Build history of the part. All positions in model axes, mm. Face numbers are marked on the shaded views. A direction names the side the tool comes from. Coordinates: 2 decimals unless noted, no trailing zeros. Order: outer loops, then holes, each group sorted by start corner. A loop starts at its lowest first (then second) coordinate and runs counter-clockwise, first axis right, second up. Notation, with made-up numbers: (43, -31) - (56, -31) arc R31 ccw to (56, -6) - close; hole circle Ø7 at (-39, -24.5). An arc over 180 degrees is marked (long way). One line per item, written item: value.
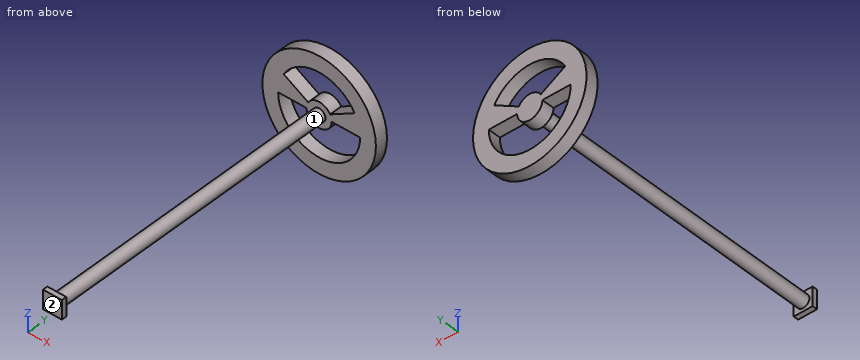
from build123d import *

# Parameters (mm, degrees)
SKETCH1_W           = 38.1
SKETCH1_H           = 38.1
BOSS_EXTRUDE1_DEPTH = 10
SKETCH2_R           = 12.7
BOSS_EXTRUDE2_DEPTH = 600
SKETCH3_R           = 114.3
BOSS_EXTRUDE3_DEPTH = 25.4
CUT_EXTRUDE2_DEPTH  = 25.4


with BuildPart() as part:
    # Sketch1 → Boss-Extrude1 (new body)
    with BuildSketch(Plane(origin=(0, 0, 0), x_dir=(1, 0, 0), z_dir=(0, 1, 0))):
        Rectangle(SKETCH1_W, SKETCH1_H)
    extrude(amount=BOSS_EXTRUDE1_DEPTH)

    # Sketch2 → Boss-Extrude2 (add)
    with BuildSketch(Plane(origin=(0, 10, 0), x_dir=(1, 0, 0), z_dir=(0, 1, 0))):
        Circle(SKETCH2_R)
    extrude(amount=BOSS_EXTRUDE2_DEPTH)

    # Sketch3 → Boss-Extrude3 (add)
    with BuildSketch(Plane(origin=(0, 610, 0), x_dir=(1, 0, 0), z_dir=(0, 1, 0))):
        Circle(SKETCH3_R)
    extrude(amount=BOSS_EXTRUDE3_DEPTH)

    # Sketch5 → Cut-Extrude2 (cut)
    with BuildSketch(Plane(origin=(0, 635.4, 0), x_dir=(1, 0, 0), z_dir=(0, 1, 0))):
        with BuildLine():
            Line((25.4, 0), (82.55, 0))
            ThreePointArc((82.55, 0), (0, 82.55), (-82.55, 0))
            Line((-82.55, 0), (-25.4, 0))
            ThreePointArc((-25.4, 0), (0, 25.4), (25.4, 0))
        make_face()
        with BuildLine():
            Line((71.490397082, -41.275), (21.997045256, -12.7))
            ThreePointArc((21.997045256, -12.7), (0, -25.4), (-21.997045256, -12.7))
            Line((-21.997045256, -12.7), (-71.490397082, -41.275))
            ThreePointArc((-71.490397082, -41.275), (0, -82.55), (71.490397082, -41.275))
        make_face()
    extrude(amount=-CUT_EXTRUDE2_DEPTH, mode=Mode.SUBTRACT)


solid = part.part
1. Flat gauge pins, fed straight in: P1, Ø8, axis at x = 4, y = 3, coming from the +Z side; P2, Ø12.5, axis at x = 45, y = 616.5, coming from the -Z side; P3, Ø11, axis at y = 6.5, z = 8.5, coming from the +X side. Where does each tip first touch, or does it go through?
Values found:
P1: stops at z = 19.05
P2: stops at z = -107.53
P3: stops at x = 19.05
2. 3-axis set-ups, long thin cutter, end or side, ignore diameter. For the marked faces 1 and 2: which of +Z, -Z, +X, -X, +Y, -Y reach the whole face in a straight line?
Values found:
face 1: none
face 2: +Z, -Z, +X, -X, -Y
3. Band-saw the part on C-C, the plane y = 164. Give the cut face in (x, z).
Values found:
outline: circle Ø25.4 at (0, 0)
4. Probe line 1 along Y through (x, z) = (-56.5, 26.5). List the from-to ranges inside material, lowest first.
Values found:
line 1: y = 610 to 635.4
5. Band-saw the part on B-B, the plane z = 34. Give the cut face in (x, y).
Values found:
outline: (-109.13, 610) - (-58.89, 610) - (-58.89, 635.4) - (-109.13, 635.4) - close; (58.89, 610) - (109.13, 610) - (109.13, 635.4) - (58.89, 635.4) - close
6. Band-saw the part on A-A, the plane x = 0. Give the cut face in (y, z).
Values found:
outline: (0, -19.05) - (10, -19.05) - (10, -12.7) - (610, -12.7) - (610, -25.4) - (635.4, -25.4) - (635.4, 25.4) - (610, 25.4) - (610, 12.7) - (10, 12.7) - (10, 19.05) - (0, 19.05) - close; (610, -114.3) - (635.4, -114.3) - (635.4, -82.55) - (610, -82.55) - close; (610, 82.55) - (635.4, 82.55) - (635.4, 114.3) - (610, 114.3) - close
7. Band-saw the part on D-D, the plane z = 72. Give the cut face in (x, y).
Values found:
outline: (-88.77, 610) - (-40.38, 610) - (-40.38, 635.4) - (-88.77, 635.4) - close; (40.38, 610) - (88.77, 610) - (88.77, 635.4) - (40.38, 635.4) - close
